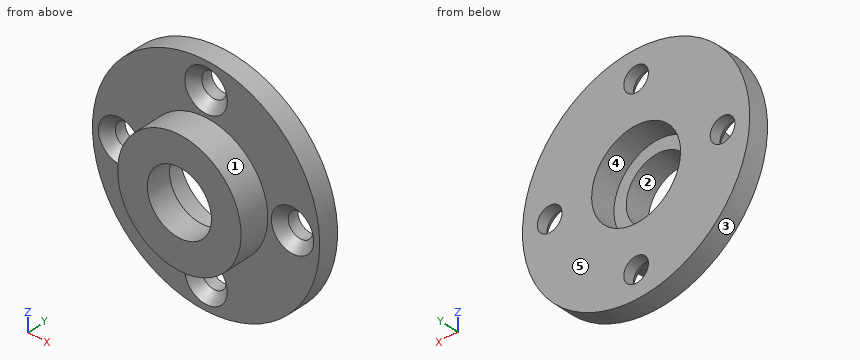
from build123d import *

# Parameters (mm, degrees)
FORO_5_0_5_1_D                        = 5
SMUSSO1_SIZE                          = 1.8
RIPETIZIONECIRCOLARE1_COUNT           = 4
SMUSSO1_OF_RIPETIZIONECIRCOLARE1_SIZE = 1.8


with BuildPart() as part:
    # Schizzo1 → Rivoluzione1 (revolve)
    with BuildSketch(Plane.XY, mode=Mode.PRIVATE) as rivoluzione1_sk:
        Polygon((6.5, 0), (12.5, 0), (12.5, 6), (23, 6), (23, 10), (9, 10), (9, 5), (6.5, 5), align=None)
    revolve(rivoluzione1_sk.sketch.rotate(Axis((0, 0, 0), (0, 1, 0)), 90), axis=Axis((0, 0, 0), (0, 1, 0)))

    # Foro Ø5.0 (5)-1 (through all)
    with Locations(Plane(origin=(0, 10, 0), x_dir=(1, 0, 0), z_dir=(0, 1, 0))):
        with Locations((17.5, 0)):
            foro_5_0_5_1 = Hole(FORO_5_0_5_1_D / 2)

    # Smusso1
    smusso1_edges = [part.edges().sort_by_distance(p)[0] for p in [
        (20, 6, 0),
    ]]
    chamfer(smusso1_edges, length=SMUSSO1_SIZE)

    # RipetizioneCircolare1: Foro Ø5.0 (5)-1 ×4 about axis
    ripetizionecircolare1_axis = Axis((0, 0, 0), (0, 1, 0))
    for i in range(1, RIPETIZIONECIRCOLARE1_COUNT):
        add(foro_5_0_5_1.rotate(ripetizionecircolare1_axis, i * 360 / RIPETIZIONECIRCOLARE1_COUNT), mode=Mode.SUBTRACT)

    # Smusso1 of RipetizioneCircolare1
    smusso1_of_ripetizionecircolare1_edges = [part.edges().sort_by_distance(p)[0] for p in [
        (0, 6, -20),
        (-20, 6, 0),
        (0, 6, 20),
    ]]
    chamfer(smusso1_of_ripetizionecircolare1_edges, length=SMUSSO1_OF_RIPETIZIONECIRCOLARE1_SIZE)


solid = part.part
Verification items for the finished model (mm, model axes). Face numbers are marked on the shaded views. A direction names the side the tool comes from. Coordinates: 2 decimals unless noted, no trailing zeros. Write each loop counter-clockwise with the first axis right and the second up, starting at its lowest first coordinate (ties: lowest second). Pieces come first, ordered by that corner, then holes. Notation, with made-up numbers: M 20,39.25 L 25,39.25 A23 cw 25,65.25 Z; hole C -38,-18.5 d1. An arc over 180 degrees is marked long. Use a Markdown table: item, result.
Q1. Sectioned sample at B-B, the plane x = 0. Record the boundary of the cut face in (y, z).
Reply:
| item | result |
|---|---|
| outline | M 0,-12.5 L 6,-12.5 L 6,-13.2 L 7.8,-15 L 10,-15 L 10,-9 L 5,-9 L 5,-6.5 L 0,-6.5 Z; M 0,6.5 L 5,6.5 L 5,9 L 10,9 L 10,15 L 7.8,15 L 6,13.2 L 6,12.5 L 0,12.5 Z; M 6,-23 L 10,-23 L 10,-20 L 7.8,-20 L 6,-21.8 Z; M 6,21.8 L 7.8,20 L 10,20 L 10,23 L 6,23 Z |
Q2. Thickness scan on line 1 (X direction, y = 1.6, z = 0); line 2 (Y direction, x = 8.5, z = 16.5); line 3 (Z direction, x = -17.5, y = 9.05). Record the ranges inside material, lowest first.
Reply:
| item | result |
|---|---|
| line 1 | x = -12.5 to -6.5, 6.5 to 12.5 |
| line 2 | y = 6 to 10 |
| line 3 | z = -14.92 to -2.5, 2.5 to 14.92 |
Q3. Go/stop test with flat-tipped pins: P1, Ø16, axis at x = 0, z = 0, coming from the -Y side; P2, Ø6, axis at x = -7, y = 5.5, coming from the +Z side; P3, Ø6, axis at x = 17.5, z = 0, coming from the -Y side; P4, Ø1.5, axis at x = 9, y = 1.5, coming from the -Z side. Record where each tip stops, or that it passes through.
Reply:
| item | result |
|---|---|
| P1 | stops at y = 0 |
| P2 | stops at z = 22.64 |
| P3 | stops at y = 7.3 |
| P4 | stops at z = -9.39 |
Q4. Sectioned sample at D-D, the plane z = -17.5. Record the boundary of the cut face in (x, y), plus the area to 3 significant figures.
Reply:
| item | result |
|---|---|
| outline | M -14.92,6 L -4.3,6 L -2.5,7.8 L -2.5,10 L -14.92,10 Z; M 2.5,7.8 L 4.3,6 L 14.92,6 L 14.92,10 L 2.5,10 Z |
| area | 96.2 mm² |
Q5. Set-up check for the marked faces 1 and 2: record each of +Z, -Z, +X, -X, +Y, -Y from which the full face is reachable in a straight line by a thin tool's end or side.
Reply:
| item | result |
|---|---|
| face 1 | -Y |
| face 2 | +Y, -Y |
Q6. Sectioned sample at A-A, the plane z = 0. Record the boundary of the cut face in (x, y), plus the area to 3 significant figures.
Reply:
| item | result |
|---|---|
| outline | M -23,6 L -21.8,6 L -20,7.8 L -20,10 L -23,10 Z; M -15,7.8 L -13.2,6 L -12.5,6 L -12.5,0 L -6.5,0 L -6.5,5 L -9,5 L -9,10 L -15,10 Z; M 6.5,0 L 12.5,0 L 12.5,6 L 13.2,6 L 15,7.8 L 15,10 L 9,10 L 9,5 L 6.5,5 Z; M 20,7.8 L 21.8,6 L 23,6 L 23,10 L 20,10 Z |
| area | 133 mm² |
Q7. Draft check along X on the marked faces 3, 4 and 5. Enter one of: +X half, -X half, draft (parallel to the pull), parting line (faces both ways), or undercut.
Reply:
| item | result |
|---|---|
| face 3 | parting line |
| face 4 | undercut |
| face 5 | draft |
Q8. Sectioned sample at C-C, the plane x = 5.5. Record the boundary of the cut face in (y, z), plus the area to 3 significant figures.
Reply:
| item | result |
|---|---|
| outline | M 0,-11.22 L 6,-11.22 L 6,-22.33 L 10,-22.33 L 10,-7.12 L 5,-7.12 L 5,-3.46 L 0,-3.46 Z; M 0,3.46 L 5,3.46 L 5,7.12 L 10,7.12 L 10,22.33 L 6,22.33 L 6,11.22 L 0,11.22 Z |
| area | 207 mm² |
